Here's how the part is built. I have some questions about the finished solid (model axes, mm). A direction names the side the tool comes from. Round coordinates to 2 decimals unless told otherwise and drop trailing zeros. Loops run counter-clockwise (first coordinate to the right, second up) from the corner with the lowest first, then second, coordinate; pieces in that order, holes last. Notation, with made-up numbers: (43.5, 82.5) - (101.5, 82.5) arc R24 cw to (101.5, 119.5) - close; hole circle Ø1 at (-16.75, -23). An arc over 180 degrees is marked (long way). Answer as a JSON object with one key per item and string values. Group by question number.
1) I want a section at A-A, the plane x = 0. Please give me the cut outline in (y, z) (3 decimals), then the cut area to 3 significant figures.
2) If we mould it in two halves opening along X, with no side actions, what happens to faces 1 (the face through (11.949, -2.056, 131.487)), 2 (the face through (0, -9.525, 40)), 3 (the face through (-12.7, 0, 40)), 4 (the face through (12.7, 0, 40))? For each: pulls with the +X half, pulls with the -X half, needs draft (parallel to the pull), parting line crosses it, or undercut.
3) I want a section at C-C, the plane y = 0. Give the number of separate pieces and of enclosed holes in the cut face, then the cut area to 3 significant figures.
4) I want a section at B-B, the plane z = 80.5. Please give me the cut outline in (x, y) (3 decimals), then the cut area to 3 significant figures.
5) Will this pin go through, and if not, where does the flat tip stop? P1, Ø5.5, axis at x = 0, z = -30.38, coming from the +Y side.
6) Which directions (+Z, -Z, +X, -X, +Y, -Y) give clear straight access to the entire face, cutting with the end or side of a thin tool? Please do faces 5 (the face through (11.949, -1.294, 106.635)), 6 (the face through (-11.176, 0, 40)).
7) If I drill on line 1 along Z through (x, y) = (0.25, 11.75); line 2 along Z through (x, y) = (0, 10.55); line 3 along Y through (x, z) = (9, -58.5) (3 decimals), over which ranges is the centre line in solid material (lowest first)? Write a range as [from, to].
from build123d import *

# Parameters (mm, degrees)
SKETCH3_W               = 25.4
SKETCH3_H               = 25.4
SKETCH3_W_2             = 22.352
SKETCH3_H_2             = 19.05
BOSS_EXTRUDE1_DEPTH     = 68.48094
FILLET1_R               = 1.6002
F_1_4_CLEARANCE_HOLE2_D = 6.7564
F_1_4_CLEARANCE_HOLE3_D = 6.7564
BOSS_EXTRUDE2_START     = 76.2
BOSS_EXTRUDE2_DEPTH     = 76.2
SKETCH17_R              = 3.3782
CUT_EXTRUDE3_DEPTH      = 148.441596571


with BuildPart() as part:
    # Sketch3 → Boss-Extrude1 (new, symmetric)
    with BuildSketch(Plane.XY):
        Rectangle(SKETCH3_W, SKETCH3_H)
        Rectangle(SKETCH3_W_2, SKETCH3_H_2, mode=Mode.SUBTRACT)
    extrude(amount=BOSS_EXTRUDE1_DEPTH, both=True)

    # Fillet1
    fillet1_edges = [part.edges().sort_by_distance(p)[0] for p in [
        (11.176, -9.525, 0),
        (11.176, 9.525, 0),
        (-11.176, 9.525, 0),
        (-11.176, -9.525, 0),
        (12.7, -12.7, 0),
        (-12.7, -12.7, 0),
        (-12.7, 12.7, 0),
        (12.7, 12.7, 0),
    ]]
    fillet(fillet1_edges, radius=FILLET1_R)

    # 1/4 Clearance Hole2 (through all)
    with Locations(Plane.ZY.offset(12.7)):
        with Locations((32.92094, 0), (45.62094, 0)):
            Hole(F_1_4_CLEARANCE_HOLE2_D / 2)

    # 1/4 Clearance Hole3 (through all)
    with Locations(Plane(origin=(0, 12.7, 0), x_dir=(1, 0, 0), z_dir=(0, 1, 0))):
        with Locations((0, 55.78094), (0, 30.38094)):
            Hole(F_1_4_CLEARANCE_HOLE3_D / 2)

    # Sketch16 → Boss-Extrude2 (add)
    with BuildSketch(Plane.XY.offset(68.48094).offset(BOSS_EXTRUDE2_START)):
        with BuildLine():
            Line((-12.7, 11.0998), (-12.7, -11.0998))
            ThreePointArc((-12.7, -11.0998), (-12.231312271, -12.231312271), (-11.0998, -12.7))
            Line((-11.0998, -12.7), (11.0998, -12.7))
            ThreePointArc((11.0998, -12.7), (12.231312271, -12.231312271), (12.7, -11.0998))
            Line((12.7, -11.0998), (12.7, 11.0998))
            ThreePointArc((12.7, 11.0998), (12.231312271, 12.231312271), (11.0998, 12.7))
            Line((11.0998, 12.7), (-11.0998, 12.7))
            ThreePointArc((-11.0998, 12.7), (-12.231312271, 12.231312271), (-12.7, 11.0998))
        make_face()
        with BuildLine():
            Line((11.176, -7.9248), (11.176, 7.9248))
            ThreePointArc((11.176, 7.9248), (10.707312271, 9.056312271), (9.5758, 9.525))
            Line((9.5758, 9.525), (-9.5758, 9.525))
            ThreePointArc((-9.5758, 9.525), (-10.707312271, 9.056312271), (-11.176, 7.9248))
            Line((-11.176, 7.9248), (-11.176, -7.9248))
            ThreePointArc((-11.176, -7.9248), (-10.707312271, -9.056312271), (-9.5758, -9.525))
            Line((-9.5758, -9.525), (9.5758, -9.525))
            ThreePointArc((9.5758, -9.525), (10.707312271, -9.056312271), (11.176, -7.9248))
        make_face(mode=Mode.SUBTRACT)
    extrude(amount=-BOSS_EXTRUDE2_DEPTH)

    # Sketch17 → Cut-Extrude3 (cut, through all)
    with BuildSketch(Plane(origin=(12.7, 0, 0), x_dir=(0, 0, -1), z_dir=(1, 0, 0))):
        with Locations((-109.75594, 0)):
            Circle(SKETCH17_R)
        with Locations((-128.80594, 0)):
            Circle(SKETCH17_R)
    extrude(amount=-CUT_EXTRUDE3_DEPTH, mode=Mode.SUBTRACT)


solid = part.part
Outcome:
{
 "1": {"outline": "(-12.7, -68.481) - (-9.525, -68.481) - (-9.525, -59.159) - (-12.7, -59.159) - close; (-12.7, -52.403) - (-9.525, -52.403) - (-9.525, -33.759) - (-12.7, -33.759) - close; (-12.7, -27.003) - (-9.525, -27.003) - (-9.525, 144.681) - (-12.7, 144.681) - close; (9.525, -68.481) - (12.7, -68.481) - (12.7, -59.159) - (9.525, -59.159) - close; (9.525, -52.403) - (12.7, -52.403) - (12.7, -33.759) - (9.525, -33.759) - close; (9.525, -27.003) - (12.7, -27.003) - (12.7, 144.681) - (9.525, 144.681) - close", "area": "1,270 mm^2"},
 "2": {"face 1": "needs draft", "face 2": "undercut", "face 3": "pulls with the -X half", "face 4": "pulls with the +X half"},
 "3": {"separate pieces": "10", "enclosed holes": "0", "area": "567 mm^2"},
 "4": {"outline": "(-12.7, -11.1) arc R1.6 ccw to (-11.1, -12.7) - (11.1, -12.7) arc R1.6 ccw to (12.7, -11.1) - (12.7, 11.1) arc R1.6 ccw to (11.1, 12.7) - (-11.1, 12.7) arc R1.6 ccw to (-12.7, 11.1) - close; hole (-11.176, -7.925) arc R1.6 ccw to (-9.576, -9.525) - (9.576, -9.525) arc R1.6 ccw to (11.176, -7.925) - (11.176, 7.925) arc R1.6 ccw to (9.576, 9.525) - (-9.576, 9.525) arc R1.6 ccw to (-11.176, 7.925) - close", "area": "219 mm^2"},
 "5": {"P1": "through"},
 "6": {"face 5": "+X, -X", "face 6": "+Z, -Z"},
 "7": {"line 1": "[-68.48, -59.15], [-52.41, -33.75], [-27.01, 144.68]", "line 2": "[-68.48, -59.16], [-52.4, -33.76], [-27, 144.68]", "line 3": "[-12.7, -9.525], [9.525, 12.7]"}
}
